Geometry: final body of the model. Coordinates: model frame, mm. Give positions to 0.01 mm unless a question says otherwise; leave off trailing zeros. Write each loop counter-clockwise with the first axis right and the second up, starting at its lowest first coordinate (ties: lowest second). Pieces come first, ordered by that corner, then holes. Notation, with made-up numbers: (19, 64) - (34, 64) arc R14 ccw to (34, 88) - close; hole circle Ø4 at (70, 87). An arc over 180 degrees is marked (long way). One line per question, with ' | ' between items. Start each with the question number.
Autodesk Inventor part; units mm, degrees
ref_plane "YZ Plane" through (0, 0, 0) normal (1, 0, 0) x (0, 1, 0)
ref_plane "XZ Plane" through (0, 0, 0) normal (0, 1, 0) x (-1, 0, 0)
ref_plane "XY Plane" through (0, 0, 0) normal (0, 0, 1) x (1, 0, 0)
sketch "Sketch1" plane through (0, 0, 0) normal (0, 1, 0) x (-1, 0, 0)
  line L0 (0, 0) -> (-4153.4811, -1112.9219) construction
  line L1 (0, 0) -> (4300, 0) construction
  line L2 (-4300, 0) -> (-4200, 0) construction
  line L3 (-2006.9086, 50) -> (-4302.025, 50)
  line L4 (-4153.4811, -1112.9219) -> (-3780.7254, -1112.9219) construction
  line L5 (-1925.5839, -567.7225) -> (-4142.0661, -1161.6271)
  line L6 (-4151.9012, -1124.9219) -> (-4302.025, 15.3817)
  line L7 (-1930.5867, -529.7225) -> (-2001.9058, 12)
  line L8 (-4263.2519, 12) -> (-2040.2337, 12)
  line L9 (-2040.2337, 12) -> (-1967.6086, -539.6424)
  line L10 (-1967.6086, -539.6424) -> (-4114.8793, -1115.0019)
  line L11 (-4114.8793, -1115.0019) -> (-4263.2519, 12)
  line L12 (-2006.9086, 50) -> (-2001.9058, 50)
  line L13 (-2040.2337, 12) -> (-1982.3344, 12) construction
  line L14 (-2001.9058, 12) -> (-2001.9058, 50)
  line L15 (-1967.6086, -539.6424) -> (-1881.5519, -516.5836) construction
  line L16 (-1930.5867, -529.7225) -> (-1920.5811, -567.0638)
  line L17 (-1920.5811, -567.0638) -> (-1925.5839, -567.7225)
  line L18 (-4263.2519, 12) -> (-4318.8305, 12) construction
  line L19 (-4302.025, 15.3817) -> (-4302.025, 50)
  line L20 (-4114.8793, -1115.0019) -> (-4170.6932, -1129.9572) construction
  line L21 (-4151.9012, -1124.9219) -> (-4142.0661, -1161.6271)
  dimension "d0" = 4300
  dimension "d1" = 4300
  dimension "d2" = 165
  dimension "d7" = 50
  dimension "d11" = 38
extrude "Extrusion2" add sketch "Sketch1" along normal blind 114
sketch "Sketch2" plane through (0, 114, 0) normal (0, 1, 0) x (1, 0, 0)
  line L0 (2040.2337, -12) -> (1967.6086, 539.6424)
  line L1 (2001.9058, -50) -> (4302.025, -50)
  line L2 (4142.0661, 1161.6271) -> (1925.5839, 567.7225)
  line L3 (1925.5839, 567.7225) -> (2001.9058, -12)
  line L4 (1967.6086, 539.6424) -> (1930.5867, 529.7225)
  line L5 (2040.2337, -12) -> (2001.9058, -12)
  point P0 (2006.9086, -50)
  point P1 (0, 0)
extrude "Extrusion3" cut sketch "Sketch2" against normal blind 1
sketch "Sketch7" plane through (0, 114, 0) normal (0, 1, 0) x (1, 0, 0)
  line L0 (4114.8793, 1115.0019) -> (4263.2519, -12)
  line L1 (4302.025, -50) -> (4302.025, -15.3817)
  line L2 (4302.025, -15.3817) -> (4151.9012, 1124.9219)
  line L3 (1920.5811, 567.0638) -> (1930.5867, 529.7225)
  line L4 (4263.2519, -12) -> (4301.5798, -12)
  line L5 (4114.8793, 1115.0019) -> (4151.9012, 1124.9219)
  point P0 (0, 0)
extrude "Extrusion6" cut sketch "Sketch7" against normal blind 1
properties part number "panelBflat" material "Wood (Birch)"
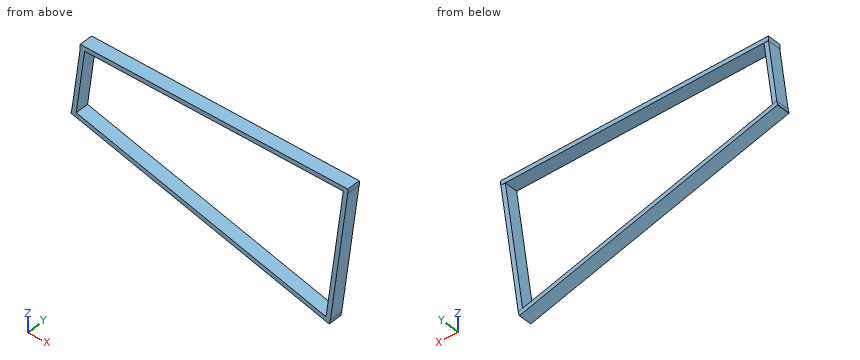
1) First-contact query: pin 1 Ø19 at (y, z) = (76.5, 24.5) entering from -X; pin 2 Ø3 at (y, z) = (44.5, -1011) entering from +X; pin 3 Ø5 at (x, y) = (2826.5, 47.5) entering from -Z. Flat tips, straight axial feed; report the tip coordinate or a pass-through.
2) Section A-A, the plane y = 60. Output: boundary loops of the cut face in (x, z) (1 decimal).
3) Section C-C, the plane z = -690.5. Output: boundary loops of the cut face in (x, y), plus the area to 3 significant figures.
4) Line query: L1, parallel to Z at x = 2111, y = 103.5; L2, parallel to Z at x = 3439, y = 70; L3, parallel to X at y = 81, z = -21. Output: solid intervals per line, ascending.
5) Section B-B, the plane x = 4023. Output: boundary loops of the cut face in (y, z).
Answer key:
1) pin 1: x = 2001.91 | pin 2: x = 4167.1 | pin 3: z = -809.79
2) outline: (1920.6, -567.1) - (1925.6, -567.7) - (4142.1, -1161.6) - (4151.9, -1124.9) - (4302, 15.4) - (4302, 50) - (2001.9, 50) - (2001.9, 12) - (1930.6, -529.7) - close; hole (1967.6, -539.6) - (4114.9, -1115) - (4263.3, 12) - (2040.2, 12) - close
3) outline: (2383.8, 0) - (2530.62, 0) - (2530.62, 114) - (2383.8, 114) - close; (4170.77, 0) - (4209.09, 0) - (4209.09, 113) - (4170.77, 113) - close | area: 21,100 mm^2
4) L1: -617.4 to -578.06, 12 to 50 | L2: -973.24 to -933.9, 12 to 50 | L3: 1997.56 to 2035.89, 4258.91 to 4297.24
5) outline: (0, -1129.72) - (114, -1129.72) - (114, -1090.38) - (0, -1090.38) - close; (0, 12) - (114, 12) - (114, 50) - (0, 50) - close
